Design review of the part built by this model. Coordinates are the model's own, in mm. Face numbers are marked on the shaded views. A direction names the side the tool comes from. Coordinates: 2 decimals unless noted, no trailing zeros. Loops run counter-clockwise (first coordinate to the right, second up) from the corner with the lowest first, then second, coordinate; pieces in that order, holes last. Notation, with made-up numbers: (50, 4.25) - (64, 4.25) arc R9 ccw to (64, 15.25) - close; hole circle Ø9 at (-5, -14.5). An arc over 180 degrees is marked (long way). One line per question, with ' | ' between items.
from build123d import *

# Parameters (mm, degrees)
SKETCH1_W           = 32
SKETCH1_H           = 60
BOSS_EXTRUDE1_DEPTH = 20
SKETCH2_R           = 7.5
SKETCH2_R_2         = 5.1
CUT_EXTRUDE1_DEPTH  = 401.819161219
SKETCH3_R           = 11
CUT_EXTRUDE2_DEPTH  = 11.75
SKETCH4_W           = 6
SKETCH4_H           = 20
BOSS_EXTRUDE2_DEPTH = 20
SKETCH5_R           = 3
CUT_EXTRUDE3_DEPTH  = 402.776057027
FILLET2_R           = 9
FILLET3_R           = 4


with BuildPart() as part:
    # Sketch1 → Boss-Extrude1 (new body)
    with BuildSketch(Plane.XY):
        with Locations((0, -370)):
            Rectangle(SKETCH1_W, SKETCH1_H)
    extrude(amount=-BOSS_EXTRUDE1_DEPTH)

    # Sketch2 → Cut-Extrude1 (cut, through all)
    with BuildSketch(Plane.XY):
        with Locations((0, -390)):
            Circle(SKETCH2_R)
        with Locations((0, -358)):
            Circle(SKETCH2_R_2)
    extrude(amount=-CUT_EXTRUDE1_DEPTH, mode=Mode.SUBTRACT)

    # Sketch3 → Cut-Extrude2 (cut)
    with BuildSketch(Plane.XY):
        with Locations((0, -358)):
            Circle(SKETCH3_R)
    extrude(amount=-CUT_EXTRUDE2_DEPTH, mode=Mode.SUBTRACT)

    # Sketch4 → Boss-Extrude2 (add)
    with BuildSketch(Plane(origin=(0, -340, 0), x_dir=(1, 0, 0), z_dir=(0, 1, 0))):
        with Locations((13, 10)):
            Rectangle(SKETCH4_W, SKETCH4_H)
        with Locations((-13, 10)):
            Rectangle(SKETCH4_W, SKETCH4_H)
    extrude(amount=BOSS_EXTRUDE2_DEPTH)

    # Sketch5 → Cut-Extrude3 (cut, through all)
    with BuildSketch(Plane.ZY.offset(16)):
        with Locations((-10.065765089, -330)):
            Circle(SKETCH5_R)
    extrude(amount=-CUT_EXTRUDE3_DEPTH, mode=Mode.SUBTRACT)

    # Fillet2
    fillet2_edges = [part.edges().sort_by_distance(p)[0] for p in [
        (16, -400, -10),
        (-16, -400, -10),
    ]]
    fillet(fillet2_edges, radius=FILLET2_R)

    # Fillet3
    fillet3_edges = [part.edges().sort_by_distance(p)[0] for p in [
        (-11, -358, 0),
    ]]
    fillet(fillet3_edges, radius=FILLET3_R)


solid = part.part
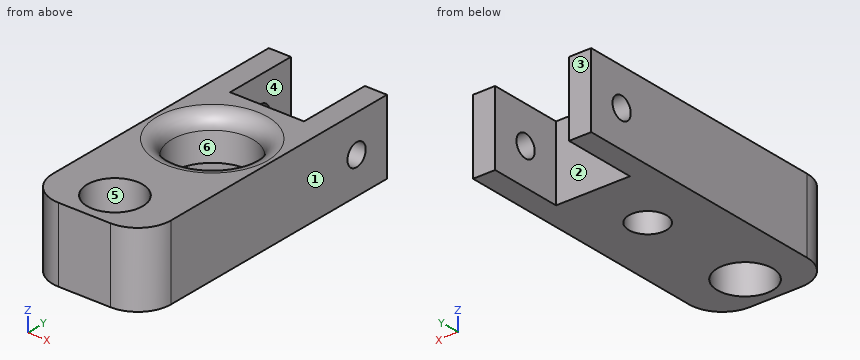
Q1. Take a section at C-C (y = -358). Give the boundary of the cut face in (x, z), plus the area to 3 significant figures.
Returned:
outline: (-16, -20) - (-5.1, -20) - (-5.1, -11.75) - (-11, -11.75) - (-11, -4) arc R4 ccw to (-15, 0) - (-16, 0) - close; (5.1, -20) - (16, -20) - (16, 0) - (15, 0) arc R4 ccw to (11, -4) - (11, -11.75) - (5.1, -11.75) - close | area: 290 mm²
Q2. For pin 1 (12 mm diameter, centred on x = -2, y = -332, fed in from -Z); pin 2 (5 mm diameter, centred on x = 5.5, z = -15, fed in from +Y); pin 3 (11 mm diameter, centred on x = 2.5, y = -357, fed in from +Z), all flat-tipped, find the tip position at first contact; note any pin that passes through.
Returned:
pin 1: passes through | pin 2: stops at y = -340 | pin 3: stops at z = -11.75
Q3. To check wall thickness, follow line 1 along Y through (x, z) = (0, -17); line 2 along Y through (x, z) = (0, -9.25); line 3 along X through (y, z) = (-358, -17). State the ranges of each line that lie inside material, in increasing order.
Returned:
line 1: y = -400 to -397.5, -382.5 to -363.1, -352.9 to -340 | line 2: y = -400 to -397.5, -382.5 to -369, -347 to -340 | line 3: x = -16 to -5.1, 5.1 to 16
Q4. Take a section at D-D (z = -10). Give the boundary of the cut face in (x, y), plus the area to 3 significant figures.
Returned:
outline: (-16, -391) arc R9 ccw to (-7, -400) - (7, -400) arc R9 ccw to (16, -391) - (16, -333) - (10, -333) - (10, -340) - (-10, -340) - (-10, -333) - (-16, -333) - close; (-16, -327) - (-10, -327) - (-10, -320) - (-16, -320) - close; (10, -327) - (16, -327) - (16, -320) - (10, -320) - close; hole circle Ø22 at (0, -358); hole circle Ø15 at (0, -390) | area: 1,500 mm²
Q5. Take a section at B-B (x = 0). Give the boundary of the cut face in (y, z).
Returned:
outline: (-400, -20) - (-397.5, -20) - (-397.5, 0) - (-400, 0) - close; (-382.5, -20) - (-363.1, -20) - (-363.1, -11.75) - (-369, -11.75) - (-369, -4) arc R4 ccw to (-373, 0) - (-382.5, 0) - close; (-352.9, -20) - (-340, -20) - (-340, 0) - (-343, 0) arc R4 ccw to (-347, -4) - (-347, -11.75) - (-352.9, -11.75) - close
Q6. Tool access review of the marked faces 4, 5 and 6: name each direction out of +Z, -Z, +X, -X, +Y, -Y from which nothing blocks a thin tool from reaching the whole face with its end or side.
Returned:
face 4: +Z, -Z, +Y | face 5: +Z, -Z | face 6: +Z
Q7. Draft analysis for pull direction X (two halves, no side actions). For the marked faces 1, 2 and 3, state which applies: +X half, -X half, draft (parallel to the pull), parting line (faces both ways), or undercut.
Returned:
face 1: +X half | face 2: undercut | face 3: draft
Q8. Take a section at A-A (y = -330). Give the boundary of the cut face in (x, z), plus the area to 3 significant figures.
Returned:
outline: (-16, -20) - (-10, -20) - (-10, -13.07) - (-16, -13.07) - close; (-16, -7.07) - (-10, -7.07) - (-10, 0) - (-16, 0) - close; (10, -20) - (16, -20) - (16, -13.07) - (10, -13.07) - close; (10, -7.07) - (16, -7.07) - (16, 0) - (10, 0) - close | area: 168 mm²
